```python
from build123d import *

# Parameters (mm, degrees)
F1_DEPTH  = 30
F2_R      = 3
F3_DEPTH  = 3.001
F5_DEPTH  = 8
F6_W      = 8
F6_H      = 2
F7_DEPTH  = 5
F8_W      = 3
F8_H      = 2
F9_DEPTH  = 4
F10_W     = 4
F10_H     = 3
F11_DEPTH = 28.001
F12_R     = 1
F13_R     = 5


with BuildPart() as f1:
    # F0 (on Front) → F1 (new body)
    with BuildSketch(Plane.XZ):
        Polygon((0, 3), (0, 0), (15, 0), (15, 34), (68, 34), (68, 0), (83, 0), (83, 3), (71, 3), (71, 37), (12, 37), (12, 3), align=None)
    extrude(amount=F1_DEPTH)

    # F2 (on face) → F3 (cut, through all)
    with BuildSketch(Plane.XY.offset(3)):
        with Locations((6, -15)):
            Circle(F2_R)
        with Locations((77, -15)):
            Circle(F2_R)
    extrude(amount=-F3_DEPTH, mode=Mode.SUBTRACT)

    # F4 (on face) → F5 (join)
    with BuildSketch(Plane.XY.offset(37)):
        Polygon((71, -30), (71, -26), (69.5, -26), (69.5, -28.5), (67, -28.5), (67, -30), align=None)
        Polygon((53.5, -6.5), (49.5, -6.5), (49.5, -10.5), (51, -10.5), (51, -8), (53.5, -8), align=None)
    extrude(amount=F5_DEPTH)

    # F6 (on face) → F7 (join)
    with BuildSketch(Plane.XY.offset(37)):
        with Locations((26, -3)):
            Rectangle(F6_W, F6_H)
        with Locations((26, -27)):
            Rectangle(F6_W, F6_H)
    extrude(amount=F7_DEPTH)

    # F8 (on face) → F9 (join)
    with BuildSketch(Plane.XY.offset(37)):
        with Locations((52.5, -9)):
            Rectangle(F8_W, F8_H)
        with Locations((68, -27.5)):
            Rectangle(F8_W, F8_H)
        with Locations((68, -9)):
            Rectangle(F8_W, F8_H)
        with Locations((52.5, -27.5)):
            Rectangle(F8_W, F8_H)
    extrude(amount=F9_DEPTH)

    # F10 (on face) → F11 (cut, through all)
    with BuildSketch(Plane.XZ.offset(28)):
        with Locations((26, 38.5)):
            Rectangle(F10_W, F10_H)
    extrude(amount=-F11_DEPTH, mode=Mode.SUBTRACT)

    # F12
    f12_edges = [f1.edges().sort_by_distance(p)[0] for p in [
        (30, -27, 42),
        (30, -3, 42),
        (22, -3, 42),
        (22, -27, 42),
        (22, -27, 37),
        (22, -3, 37),
        (29, -4, 37),
        (23, -4, 37),
        (30, -3, 37),
        (29, -28, 37),
        (23, -28, 37),
        (30, -27, 37),
        (29, -26, 37),
        (23, -26, 37),
        (29, -2, 37),
        (23, -2, 37),
        (51.5, -6.5, 37),
        (49.5, -8.5, 37),
        (50.25, -10.5, 37),
    ]]
    fillet(f12_edges, radius=F12_R)

    # F13
    f13_edges = [f1.edges().sort_by_distance(p)[0] for p in [
        (83, -30, 1.5),
        (83, 0, 1.5),
        (0, 0, 1.5),
        (0, -30, 1.5),
    ]]
    fillet(f13_edges, radius=F13_R)


solid = f1.part
```
Geometry: final body of the model. Coordinates: model frame, mm. A direction names the side the tool comes from. Round coordinates to 2 decimals unless told otherwise and drop trailing zeros. Order: outer loops, then holes, each group sorted by start corner. A loop starts at its lowest first (then second) coordinate and runs counter-clockwise, first axis right, second up. Notation, with made-up numbers: (-26.75, 67.5) - (15.25, 67.5) arc R8 ccw to (15.25, 72.5) - close; hole circle Ø11 at (-26.5, 20). An arc over 180 degrees is marked (long way). Use CSV: the item, a comma, the result in double quotes. Start each with the question number.
Q1. Access query for faces 4 (the face through (28, -27, 38)), 5 (the face through (22, -27, 39)), 6 (the face through (15, -15, 17)). Directions: +Z, -Z, +X, -X, +Y, -Y. A direction counts if a zero-diameter tool reaches every point of the face in a straight line with its end or side. Return the directions, or none.
Q2. Section query B-B (x = 6). Return loops of the section in (y, z), and give its area (3 significant figures).
Q3. Section query D-D (y = -21.5). Return loops of the section in (x, z).
Q4. Section query A-A (y = -15). Return loops of the section in (x, z), and give its area (3 significant figures).
Q5. Material intervals for line 1 along Y through (x, z) = (6, 1); line 2 along X through (y, z) = (-27.75, 21); line 3 along Z through (x, y) = (25, -2.75), sorted ascending. Write a range as from..to.
Q6. First-contact query: pin 1 (1 mm diameter, centred on y = -8.5, z = 39, fed in from -X); pin 2 (8 mm diameter, centred on x = 6, y = -15, fed in from +Z); pin 3 (3 mm diameter, centred on x = 52, z = 43.5, fed in from -Y). Flat tips, straight axial feed; report the tip coordinate or a pass-through.
Q7. Section query C-C (z = 21). Return loops of the section in (x, y), and give its area (3 significant figures).
Q8. Mould query, pull axis Z, two halves, no side actions, for faces 1 (the face through (50.6, -8, 45)), 2 (the face through (26, -27, 40)), 3 (the face through (82, -28, 2)). Classes: +Z half, -Z half, draft (parallel to the pull), parting line (faces both ways), or undercut.
Result set:
1,face 4,"+Y, -Y"
1,face 5,"+Z, -X, +Y, -Y"
1,face 6,"-Z, +Y, -Y"
2,outline,"(-30, 0) - (-18, 0) - (-18, 3) - (-30, 3) - close; (-12, 0) - (0, 0) - (0, 3) - (-12, 3) - close"
2,area,"72.0 mm2"
3,outline,"(0, 0) - (15, 0) - (15, 34) - (68, 34) - (68, 0) - (83, 0) - (83, 3) - (71, 3) - (71, 37) - (12, 37) - (12, 3) - (0, 3) - close"
4,outline,"(0, 0) - (3, 0) - (3, 3) - (0, 3) - close; (9, 0) - (15, 0) - (15, 34) - (68, 34) - (68, 0) - (74, 0) - (74, 3) - (71, 3) - (71, 37) - (12, 37) - (12, 3) - (9, 3) - close; (80, 0) - (83, 0) - (83, 3) - (80, 3) - close"
4,area,"417 mm2"
5,line 1,"y = -30..-18, -12..0"
5,line 2,"x = 12..15, 68..71"
5,line 3,"z = 34..37, 40..42"
6,pin 1,"stops at x = 49.5"
6,pin 2,"stops at z = 3"
6,pin 3,"stops at y = -10.5"
7,outline,"(12, -30) - (15, -30) - (15, 0) - (12, 0) - close; (68, -30) - (71, -30) - (71, 0) - (68, 0) - close"
7,area,"180 mm2"
8,face 1,"+Z half"
8,face 2,"undercut"
8,face 3,"draft"
